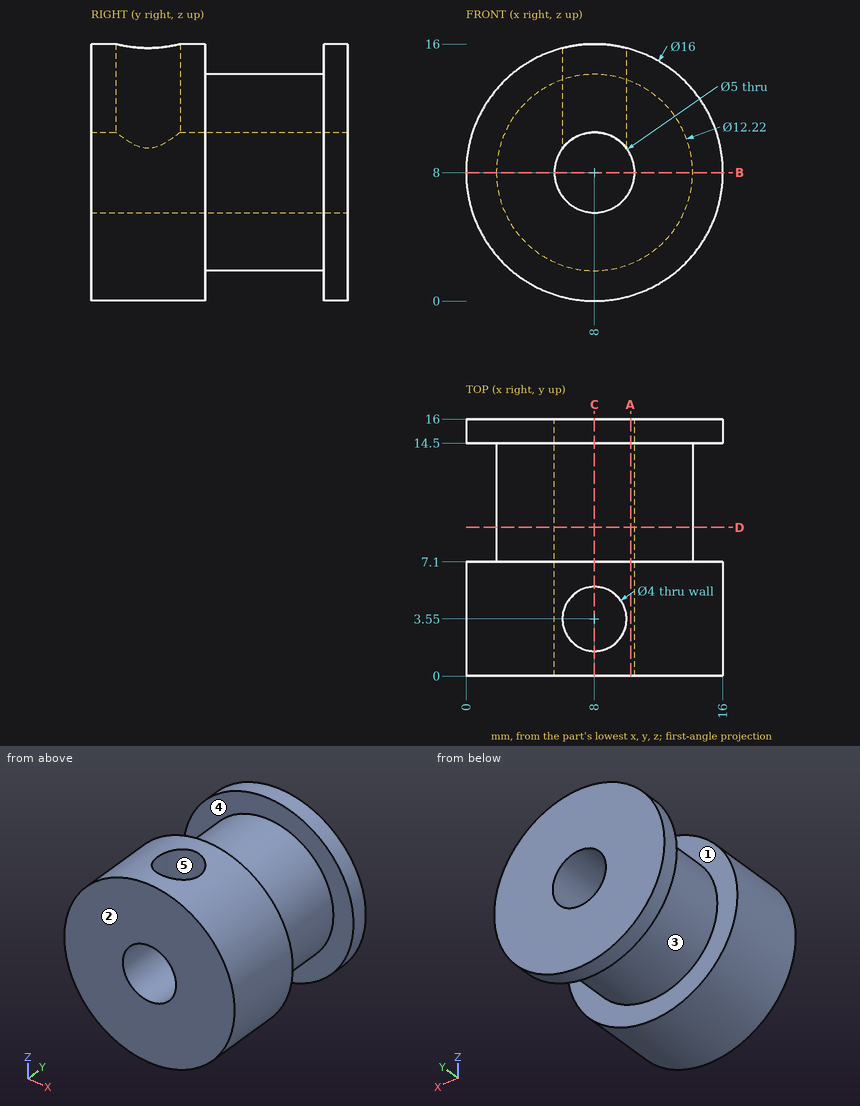
Drawing for the job (mm, zero at the part's lowest x, y, z). A direction names the side the tool comes from. Round coordinates to 2 decimals unless told otherwise and drop trailing zeros. Loops run counter-clockwise (first coordinate to the right, second up) from the corner with the lowest first, then second, coordinate; pieces in that order, holes last. Notation, with made-up numbers: M -16.5,38.25 L 17.5,38.25 A22 ccw 17.5,47.25 Z; hole C -32,-19.75 d5. An arc over 180 degrees is marked long. Use a Markdown table: item, result. Add a question column.
(1) Pull direction X, two halves, no side cores. Call the marked faces 3, 4 and 5: +X half, -X half, draft (parallel to the pull), parting line (faces both ways), or undercut.
(2) Cut at A-A (x = 10.25). Give the cut face in (y, z).
(3) Which spindle directions (+Z, -Z, +X, -X, +Y, -Y) get a long thin tool onto all of the face, cutting with end or side? Do the marked faces 1 and 2. Say none if no direction does.
(4) Cut at D-D (y = 9.25). Give the cut face in (x, z).
(5) Drill centre lines: line 1 (Y direction, x = 13.75, z = 10.5); line 2 (Y direction, x = 8, z = 12.25); line 3 (Y direction, x = 8, z = 14.5). Where is each one in solid material? Low to high.
(6) Flat gauge pins, fed straight in: pin 1 (5 mm diameter, centred on x = 12.5, y = 10.5, fed in from -Z); pin 2 (4 mm diameter, centred on y = 5.5, z = 5, fed in from -X); pin 3 (2.5 mm diameter, centred on x = 8, y = 3.55, fed in from +Z). Where does each tip first touch, or does it go through?
(7) Cut at B-B (z = 8). Give the cut face in (x, y), and give its area (3 significant figures).
(8) Cut at C-C (x = 8). Give the cut face in (y, z), and give its area (3 significant figures).
Geometry says:
| question | item | result |
|---|---|---|
| 1 | face 3 | parting line |
| 1 | face 4 | draft |
| 1 | face 5 | undercut |
| 2 | outline | M 0,0.32 L 7.1,0.32 L 7.1,2.32 L 14.5,2.32 L 14.5,0.32 L 16,0.32 L 16,6.91 L 0,6.91 Z; M 0,9.09 L 16,9.09 L 16,15.68 L 14.5,15.68 L 14.5,13.68 L 7.1,13.68 L 7.1,15.68 L 0,15.68 Z |
| 3 | face 1 | none |
| 3 | face 2 | +Z, -Z, +X, -X, -Y |
| 4 | outline | C 8,8 d12.22; hole C 8,8 d5 |
| 5 | line 1 | y = 0 to 7.1, 14.5 to 16 |
| 5 | line 2 | y = 0 to 1.55, 5.55 to 16 |
| 5 | line 3 | y = 0 to 1.55, 5.55 to 7.1, 14.5 to 16 |
| 6 | pin 1 | stops at z = 2.23 |
| 6 | pin 2 | stops at x = 0.06 |
| 6 | pin 3 | stops at z = 5.83 |
| 7 | outline | M 0,0 L 5.5,0 L 5.5,16 L 0,16 L 0,14.5 L 1.89,14.5 L 1.89,7.1 L 0,7.1 Z; M 10.5,0 L 16,0 L 16,7.1 L 14.11,7.1 L 14.11,14.5 L 16,14.5 L 16,16 L 10.5,16 Z |
| 7 | area | 148 mm² |
| 8 | outline | M 0,0 L 7.1,0 L 7.1,1.89 L 14.5,1.89 L 14.5,0 L 16,0 L 16,5.5 L 0,5.5 Z; M 0,10.5 L 1.55,10.5 L 1.55,16 L 0,16 Z; M 5.55,10.5 L 16,10.5 L 16,16 L 14.5,16 L 14.5,14.11 L 7.1,14.11 L 7.1,16 L 5.55,16 Z |
| 8 | area | 126 mm² |
